Part print with two shaded views. Sizes in mm from the minimum x, y, z corner. A direction names the side the tool comes from. Coordinates: 2 decimals unless noted, no trailing zeros. Loops run counter-clockwise (first coordinate to the right, second up) from the corner with the lowest first, then second, coordinate; pieces in that order, holes last. Notation, with made-up numbers: (-9, -28.75) - (14, -28.75) arc R19 cw to (14, -21.75) - close; hole circle Ø10 at (53.5, 70.5). An arc over 180 degrees is marked (long way). Answer as CSV lines item,"result".
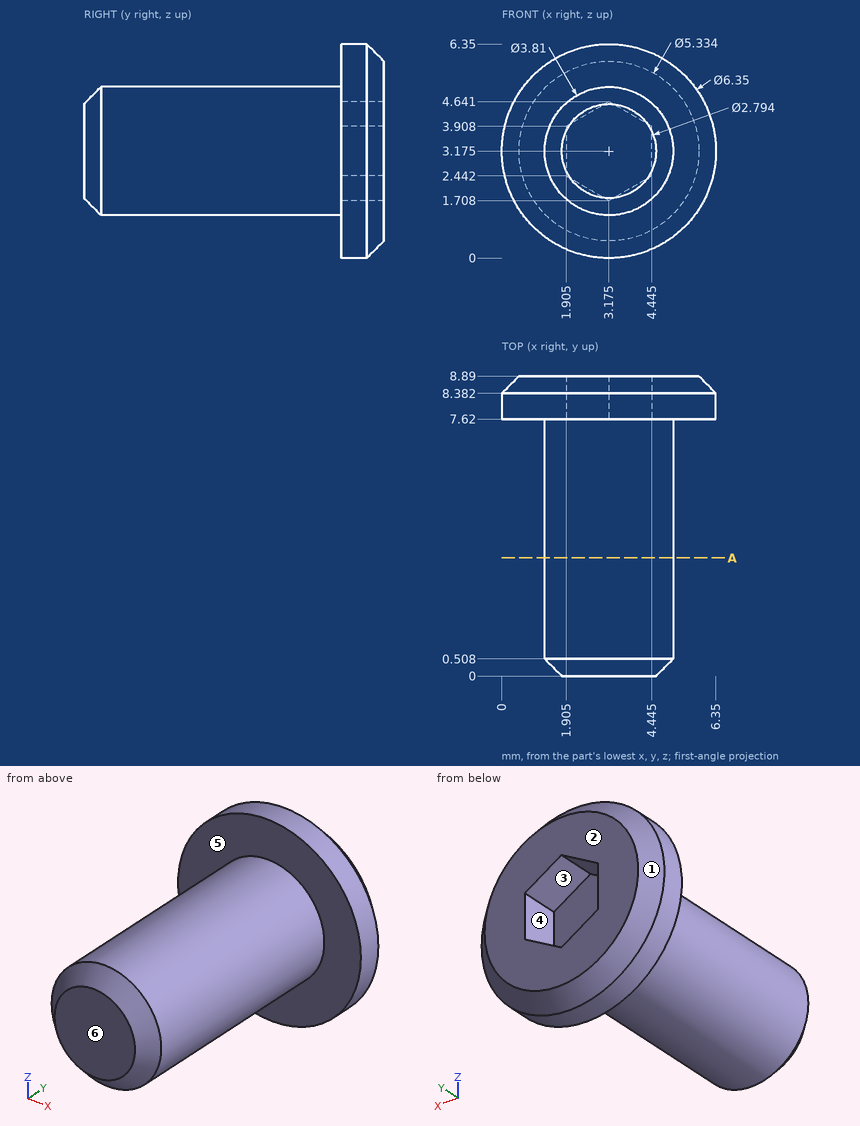
Q1. Two-plate mould, pull along Z, no slides. Class the marked faces 1, 2 and 3: released by +Z, released by -Z, zero draft, split by the parting line, or undercut.
Results:
face 1,"split by the parting line"
face 2,"zero draft"
face 3,"undercut"
Q2. Saw through at A-A (y = 3.5). Give the cut face in (x, z) (1 decimal).
Results:
outline,"circle Ø3.8 at (3.2, 3.2)"
Q3. Which spindle directions (+Z, -Z, +X, -X, +Y, -Y) get a long thin tool onto all of the face, cutting with end or side? Do the marked faces 4, 5 and 6. Say none if no direction does.
Results:
face 4,"+Y"
face 5,"-Y"
face 6,"+Z, -Z, +X, -X, -Y"
Q4. Flat gauge pin, fed straight in: pin 1 (0.8 mm diameter, centred on x = 3.5, z = 2.5, fed in from +Y). Where does the tip first touch, or does it go through?
Results:
pin 1,"stops at y = 7.62"
Q5. Wall check: L1, parallel to Y at x = 4, z = 2.75; L2, parallel to Z at x = 2, y = 8.25 (1 decimal); L3, parallel to Z at x = 3.25, y = 4.5. Give the ranges that are in metal, low to high.
Results:
L1,"y = 0 to 7.62"
L2,"z = 0.2 to 2.4, 4 to 6.1"
L3,"z = 1.27 to 5.08"
